```python
from build123d import *

# Parameters (mm, degrees)
SKETCH1_R                     = 9
BOSS_EXTRUDE1_DEPTH           = 29
BOSS_EXTRUDE1_TAPER           = 2
BOSS_EXTRUDE1_OTHER_WAY_DEPTH = 6
BOSS_EXTRUDE1_OTHER_WAY_TAPER = -2
CUT_EXTRUDE1_DEPTH            = 32.790418169
CUT_EXTRUDE1_DEPTH_BACK       = 32.790418169
CUT_EXTRUDE2_START            = -10.365035118
CUT_EXTRUDE2_OUTLINE_W        = 9.770566763
CUT_EXTRUDE2_OUTLINE_H        = 6
CUT_EXTRUDE2_DEPTH            = 10.365035118
CUT_EXTRUDE3_DEPTH            = 34.493511964
CUT_EXTRUDE3_DEPTH_BACK       = 34.493511964
SKETCH5_R                     = 1.5
FILLET1_SIZE                  = 5
CUT_EXTRUDE4_DEPTH            = 32.730353664
CUT_EXTRUDE4_DEPTH_BACK       = 32.730353664
SKETCH8_W                     = 10
SKETCH8_H                     = 6
CUT_EXTRUDE5_DEPTH            = 33.084793141
CUT_EXTRUDE6_DEPTH            = 34.493511964
CUT_EXTRUDE6_DEPTH_BACK       = 34.493511964
SKETCH9_R                     = 1.5
FILLET2_SIZE                  = 5
CUT_EXTRUDE7_DEPTH            = 38.293636915


with BuildPart() as part:
    # Sketch1 → Boss-Extrude1 (new body)
    with BuildSketch(Plane(origin=(0, 0, 0), x_dir=(1, 0, 0), z_dir=(0, 1, 0))):
        Circle(SKETCH1_R)
    extrude(amount=BOSS_EXTRUDE1_DEPTH, taper=BOSS_EXTRUDE1_TAPER)

    # Sketch1 → Boss-Extrude1 other way (add)
    with BuildSketch(Plane(origin=(0, 0, 0), x_dir=(1, 0, 0), z_dir=(0, 1, 0))):
        Circle(SKETCH1_R)
    extrude(amount=-BOSS_EXTRUDE1_OTHER_WAY_DEPTH, taper=BOSS_EXTRUDE1_OTHER_WAY_TAPER)

    # Sketch3 → Cut-Extrude1 (cut, two sides: drawn at the far end of the back side and taken through both)
    with BuildSketch(Plane(origin=(0, 0, 0), x_dir=(0, 0, -1), z_dir=(1, 0, 0)).offset(-CUT_EXTRUDE1_DEPTH_BACK)):
        Polygon((-1.155510401, -6), (-1.155510401, 0), (-11.155510401, 10), (-11.155510401, -6), align=None)
    extrude(amount=CUT_EXTRUDE1_DEPTH + CUT_EXTRUDE1_DEPTH_BACK, mode=Mode.SUBTRACT)

    # Cut-Extrude2: read off the stored shape, not the designer's step
    # Cut-Extrude2 outline → Cut-Extrude2 (cut)
    with BuildSketch(Plane.XY.offset(1.155510401).offset(CUT_EXTRUDE2_START)):
        with Locations((-9.885283382, -3)):
            Rectangle(CUT_EXTRUDE2_OUTLINE_W, CUT_EXTRUDE2_OUTLINE_H)
        with Locations((9.885283382, -3)):
            Rectangle(CUT_EXTRUDE2_OUTLINE_W, CUT_EXTRUDE2_OUTLINE_H)
    extrude(amount=CUT_EXTRUDE2_DEPTH, mode=Mode.SUBTRACT)

    # Sketch5 → Cut-Extrude3 (cut, two sides: drawn at the far end of the back side and taken through both)
    with BuildSketch(Plane.ZY.offset(5).offset(-CUT_EXTRUDE3_DEPTH_BACK)):
        with Locations(Location((-1.344489599, -3.5, 0), (0, 0, 270))):
            Circle(SKETCH5_R)
    extrude(amount=CUT_EXTRUDE3_DEPTH + CUT_EXTRUDE3_DEPTH_BACK, mode=Mode.SUBTRACT)

    # Fillet1
    # a fillet whose section is not a circle: 5 mm, written as the material it takes off along each edge
    with BuildSketch(Plane(origin=(17.5, -6, 1.155510401), x_dir=(0, 0, -1), z_dir=(-1, 0, 0))) as fillet1_piece_1:
        with BuildLine():
            Bezier((FILLET1_SIZE, 0), (0, 0), (0, -FILLET1_SIZE), weights=[1, 1.5, 1])
            Line((0, -FILLET1_SIZE), (0, 0))
            Line((0, 0), (FILLET1_SIZE, 0))
        make_face()
    extrude(amount=35, mode=Mode.SUBTRACT)

    # Sketch7 → Cut-Extrude4 (cut, two sides: drawn at the far end of the back side and taken through both)
    with BuildSketch(Plane(origin=(0, 0, 0), x_dir=(0, 0, -1), z_dir=(1, 0, 0)).offset(-CUT_EXTRUDE4_DEPTH_BACK)):
        Polygon((-1.155510401, 29), (-1.155510401, 23), (-12.24506556, 11.91044484), (-12.24506556, 29), align=None)
    extrude(amount=CUT_EXTRUDE4_DEPTH + CUT_EXTRUDE4_DEPTH_BACK, mode=Mode.SUBTRACT)

    # Sketch8 → Cut-Extrude5 (cut, through all)
    with BuildSketch(Plane.XY.offset(1.155510401)):
        with Locations((0, 26)):
            Rectangle(SKETCH8_W, SKETCH8_H)
    extrude(amount=-CUT_EXTRUDE5_DEPTH, mode=Mode.SUBTRACT)

    # Sketch9 → Cut-Extrude6 (cut, two sides: drawn at the far end of the back side and taken through both)
    with BuildSketch(Plane(origin=(-5, 0, 0), x_dir=(0, 0, -1), z_dir=(1, 0, 0)).offset(-CUT_EXTRUDE6_DEPTH_BACK)):
        with Locations(Location((1.344489599, 26.5, 0), (0, 0, 298.528207369))):
            Circle(SKETCH9_R)
    extrude(amount=CUT_EXTRUDE6_DEPTH + CUT_EXTRUDE6_DEPTH_BACK, mode=Mode.SUBTRACT)

    # Fillet2
    # a fillet whose section is not a circle: 5 mm, written as the material it takes off along each edge
    with BuildSketch(Plane(origin=(-20.403272741, 29, 1.155510401), x_dir=(0, 0, -1), z_dir=(1, 0, 0))) as fillet2_piece_1:
        with BuildLine():
            Bezier((FILLET2_SIZE, 0), (0, 0), (0, -FILLET2_SIZE), weights=[1, 1.5, 1])
            Line((0, -FILLET2_SIZE), (0, 0))
            Line((0, 0), (FILLET2_SIZE, 0))
        make_face()
    extrude(amount=27.903272741, mode=Mode.SUBTRACT)
    with BuildSketch(Plane(origin=(-7.5, 29, 1.155510401), x_dir=(0, -1, 0), z_dir=(1, 0, 0))) as fillet2_piece_2:
        with BuildLine():
            Bezier((FILLET2_SIZE, 0), (0, 0), (0, FILLET2_SIZE), weights=[1, 1.5, 1])
            Line((0, FILLET2_SIZE), (0, 0))
            Line((0, 0), (FILLET2_SIZE, 0))
        make_face()
    extrude(amount=27.903272741, mode=Mode.SUBTRACT)

    # Sketch10 → Cut-Extrude7 (cut, through all)
    with BuildSketch(Plane.XZ.offset(6)):
        with BuildLine():
            Line((-4, -3.844489599), (-4, -5.998103467))
            ThreePointArc((-4, -5.998103467), (0, -7.209524617), (4, -5.998103467))
            Line((4, -5.998103467), (4, -3.844489599))
            Line((4, -3.844489599), (-4, -3.844489599))
        make_face()
    extrude(amount=-CUT_EXTRUDE7_DEPTH, mode=Mode.SUBTRACT)


solid = part.part
```
Check sheet for the modelled part. Datum: model origin and axes. Units: mm. A direction names the side the tool comes from. Give positions to 0.01 mm unless a question says otherwise; leave off trailing zeros. Order: outer loops, then holes, each group sorted by start corner. A loop starts at its lowest first (then second) coordinate and runs counter-clockwise, first axis right, second up. Notation, with made-up numbers: (-35, 57) -> (-1, 57) arc R24 ccw to (-1, 74) -> close; hole circle Ø1 at (71.5, 62). An arc over 180 degrees is marked (long way). Return JSON: item names as keys, results as strings.
1. Mould release check, pull along Z, two halves, no side actions. Record for faces 4 (the cylindrical face through (-6.6, 26.1, 0.1)), 5 (the flat face through (5, 26, -3)), 6 (the flat face through (-0.114, 20.214, 3.942)), 7 (the flat face through (-4, 8, -5)): +Z half, -Z half, draft (parallel to the pull), parting line (faces both ways), or undercut.
From the geometry:
{"face 4": "undercut", "face 5": "draft", "face 6": "+Z half", "face 7": "undercut"}
2. Cross-section at A-A, the plane y = -3.5. Count the separate pieces of the cut face and the enclosed holes in it, plus the area to 3 significant figures.
From the geometry:
{"separate pieces": "2", "enclosed holes": "1", "area": "41.9 mm^2"}
3. Go/stop test with flat-tipped pins: P1, Ø5, axis at y = 26.5, z = -1, coming from the -X side; P2, Ø2, axis at x = 7, z = -3, coming from the -Y side; P3, Ø1.5, axis at x = 2.5, z = -4, coming from the +Y side; P4, Ø1.8, axis at y = -3.5, z = -1.34, coming from the +X side. Record where each tip stops, or that it passes through.
From the geometry:
{"P1": "x = -8.16", "P2": "y = 0", "P3": "y = 23", "P4": "through"}
4. Material ranges on probe 1 along Z at (x, y) = (-2, -3.5); probe 2 along X at (y, z) = (2, -6.25); probe 3 along X at (y, z) = (7.5, -5.25), recorded low to high. Write a range as [from, to].
From the geometry:
{"probe 1": "[-8.9, -6.93], [-3.84, -2.84], [0.16, 0.93]", "probe 2": "[-6.38, -3.59], [3.59, 6.38]", "probe 3": "[-6.99, -4], [4, 6.99]"}
5. Cross-section at B-B, the plane y = 3. Record the cut outline in (x, z).
From the geometry:
{"outline": "(-7.86, 4.16) arc R8.9 ccw (long way) to (7.86, 4.16) -> close; hole (-4, -6) arc R7.21 ccw to (4, -6) -> (4, -3.84) -> (-4, -3.84) -> close"}
6. Set-up check for faces 1 (the flat face through (5, -3, -4)), 2 (the flat face through (-0.1, -0.5, 1.156)), 3 (the cylindrical face through (-0.06, 8.3, -7.21)): record each of +Z, -Z, +X, -X, +Y, -Y from which the full face is reachable in a straight line by a thin tool's end or side.
From the geometry:
{"face 1": "+Z, -Z, +X, -Y", "face 2": "+Z, +X, -X, -Y", "face 3": "+Y, -Y"}
